Answer from the drawing. Dimensions are ordinates in mm from the lowest x, y and z of the part. A direction names the side the tool comes from. Give positions to 0.01 mm unless a question says otherwise; leave off trailing zeros. Order: outer loops, then holes, each group sorted by start corner. A loop starts at its lowest first (then second) coordinate and runs counter-clockwise, first axis right, second up.
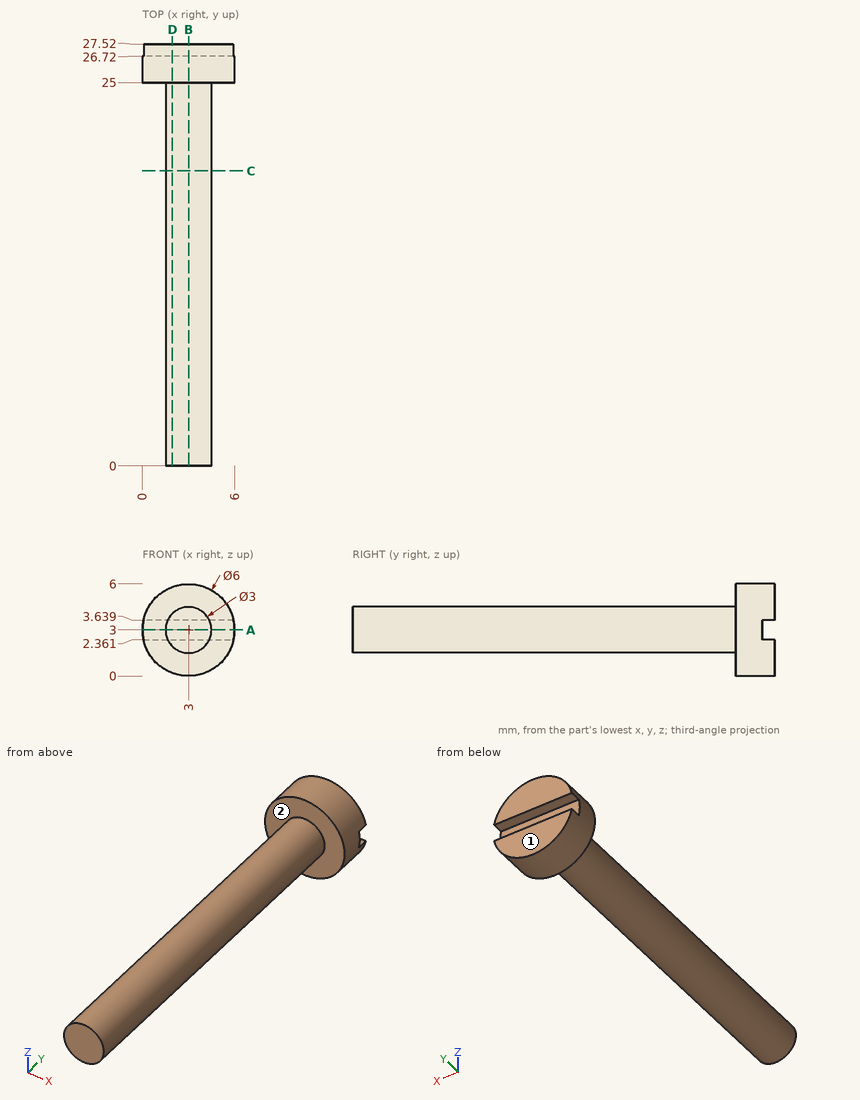
1) Consider L1, parallel to Y at x = 1.3, z = 4.95; L2, parallel to Y at x = 2.6, z = 2.8; L3, parallel to X at y = 22.5, z = 2.4 (1 decimal). Determine where each line is inside the solid, lowest interval first.
Final values:
L1: y = 25 to 27.52
L2: y = 0 to 26.72
L3: x = 1.6 to 4.4
2) The part is cut by section B-B on x = 3. Determine the outline of the cut face in (y, z).
Final values:
outline: (0, 1.5) - (25, 1.5) - (25, 0) - (27.52, 0) - (27.52, 2.36) - (26.72, 2.36) - (26.72, 3.64) - (27.52, 3.64) - (27.52, 6) - (25, 6) - (25, 4.5) - (0, 4.5) - close
3) The part is cut by section A-A on z = 3. Determine the outline of the cut face in (x, y).
Final values:
outline: (0, 25) - (1.5, 25) - (1.5, 0) - (4.5, 0) - (4.5, 25) - (6, 25) - (6, 26.72) - (0, 26.72) - close
4) The part is cut by section C-C on y = 19.25. Determine the outline of the cut face in (x, z).
Final values:
outline: circle Ø3 at (3, 3)
5) The part is cut by section D-D on x = 1.95. Determine the outline of the cut face in (y, z).
Final values:
outline: (0, 1.93) - (25, 1.93) - (25, 0.19) - (27.52, 0.19) - (27.52, 2.36) - (26.72, 2.36) - (26.72, 3.64) - (27.52, 3.64) - (27.52, 5.81) - (25, 5.81) - (25, 4.07) - (0, 4.07) - close
6) Given pin 1 (1 mm diameter, centred on x = 4, y = 20.5, fed in from +Z); pin 2 (0.6 mm diameter, centred on x = 3.5, y = 27, fed in from -Z); pin 3 (3 mm diameter, centred on y = 5.5, z = 1.5, fed in from +X); pin 4 (3 mm diameter, centred on x = 3.5, z = 2, fed in from -Y), each flat-ended and moving along its own axis, determine where each tip first touches the part or whether it passes through.
Final values:
pin 1: stops at z = 4.41
pin 2: stops at z = 0.01
pin 3: stops at x = 4.5
pin 4: stops at y = 0
7) A tool of negligible diameter and unlimited length cuts with its end or side. For the marked faces 1 and 2, from which of +Z, -Z, +X, -X, +Y, -Y can it reach the whole face along a straight path? Write none if from no direction.
Final values:
face 1: +Z, -Z, +X, -X, +Y
face 2: -Y
